CAD build for the part. Positions are in the model's coordinates, mm. A direction names the side the tool comes from. Give positions to 0.01 mm unless a question says otherwise; leave off trailing zeros. Write each loop counter-clockwise with the first axis right and the second up, starting at its lowest first coordinate (ties: lowest second). Pieces come first, ordered by that corner, then holes. Notation, with made-up numbers: (-32.5, 56.5) - (-15.5, 56.5) arc R23 ccw to (-15.5, 78.5) - close; hole circle Ø10 at (28.25, -30.5). An arc over 180 degrees is marked (long way). Put each result on its own line as item: value. Start each with the question number.
1. Tool access for faces 1 (the flat face through (1, 3.175, 4)), 2 (the flat face through (3, 2, 285)): list every direction of +Z, -Z, +X, -X, +Y, -Y with a clear straight run to the whole face (end or side of a thin tool).
2. Wall check: line 1 (Y direction, x = 94, z = 177) (3 decimals); line 2 (X direction, y = 8.25, z = 122) (3 decimals); line 3 (X direction, y = 5.75, z = 253.5). Give the ranges that are in metal, low to high.
3. Cut at A-A on z = 11.5. List the corners of the cut face in (x, y) (3 decimals), and give its area (3 significant figures).
4. Cut at B-B on x = 38.5. List the corners of the cut face in (y, z) (3 decimals), and give its area (3 significant figures).
5. Drop flat-ended pins along their axis: pin 1 (8 mm diameter, centred on x = -60.5, z = 224.5, fed in from +Y) (3 decimals); pin 2 (1.1 mm diameter, centred on y = 8.5, z = 28, fed in from -X) (3 decimals); pin 3 (1.5 mm diameter, centred on y = 6.5, z = 166.5, fed in from -X); pin 4 (1 mm diameter, centred on x = -65, y = 5.5, fed in from -Z). Give the stop position or say it passes through.
Autodesk Inventor part; units mm, degrees
ref_plane "YZ Plane" through (0, 0, 0) normal (1, 0, 0) x (0, 1, 0)
ref_plane "XZ Plane" through (0, 0, 0) normal (0, 1, 0) x (-1, 0, 0)
ref_plane "XY Plane" through (0, 0, 0) normal (0, 0, 1) x (1, 0, 0)
sketch "Sketch1" plane through (0, 0, 0) normal (0, 1, 0) x (-1, 0, 0)
  line L0 (97, 285) -> (-97, 285)
  line L1 (-97, 285) -> (-97, -285)
  line L2 (-97, -285) -> (97, -285)
  line L3 (97, -285) -> (97, 285)
  point P0 (0, 0)
  dimension "d0" = 194
  dimension "d1" = 570
  dimension "d2" = 97
  dimension "d3" = 285
extrude "Plate1" add sketch "Sketch1" along normal blind 3.175
sketch "Sketch3" plane through (100.175, 6.35, -285) normal (1, 0, 0) x (0, 1, 0)
  line L0 (0, 570) -> (0, 0)
  line L1 (0, 0) -> (3.65, 0)
  line L2 (3.65, 0) -> (3.65, 570)
  line L3 (3.65, 570) -> (0, 570)
edge flange "Flange1" height 10 angle 90 thickness 3.175 bend radius 3.175 thickness toward (1, 0, 0) relief tear relief width 3.175 relief depth 1.5875 edges at (97, 3.175, 0) wall of the first edge with corners at (100.175, 6.35, 285) (100.175, 6.35, -285) (100.175, 10, -285) (100.175, 10, 285)
bend "Bend1"
corner "Corner1"
equation "\"d4\" = Thickness"
equation "\"d5\" = BendReliefWidth"
equation "\"d6\" = BendReliefDepth"
equation "\"d7\" = MinimumRemnant"
equation "\"d8\" = TransitionRadius"
equation "\"d11\" = BendRadius"
equation "\"d12\" = CornerReliefSize"
equation "\"d13\" = GapSize"
equation "\"d14\" = JacobiRadiusSize"
equation "\"BendRadius\" = Thickness"
equation "\"BendReliefWidth\" = Thickness"
equation "\"BendReliefDepth\" = 0.5 * Thickness"
equation "\"CornerReliefSize\" = 4 * Thickness"
equation "\"MinimumRemnant\" = 2 * Thickness"
equation "\"TransitionRadius\" = BendRadius"
equation "\"JacobiRadiusSize\" = BendRadius"
equation "\"GapSize\" = Thickness"
properties part number "CO-1-01-controlsSeperator"
Report:
1. face 1: +Z, -Z, -X, +Y
1. face 2: +Z, +X, -X, +Y, -Y
2. line 1: y = 0 to 3.175
2. line 2: x = 100.175 to 103.35
2. line 3: x = 100.12 to 103.32
3. outline: (-97, 0) - (97, 0) arc R6.35 ccw to (103.35, 6.35) - (103.35, 10) - (100.175, 10) - (100.175, 6.35) arc R3.175 cw to (97, 3.175) - (-97, 3.175) - close
3. area: 651 mm²
4. outline: (0, -285) - (3.175, -285) - (3.175, 285) - (0, 285) - close
4. area: 1,810 mm²
5. pin 1: stops at y = 3.175
5. pin 2: stops at x = 100.175
5. pin 3: stops at x = 100.12
5. pin 4: passes through
